Could you check a few things on this model? Use its own coordinates, in mm. A direction names the side the tool comes from. Coordinates: 2 decimals unless noted, no trailing zeros. Write each loop counter-clockwise with the first axis right and the second up, starting at its lowest first coordinate (ties: lowest second). Pieces come first, ordered by that corner, then holes. Notation, with made-up numbers: (50.5, 52.5) - (105.5, 52.5) arc R22 cw to (105.5, 86.5) - close; hole circle Ø2 at (58.5, -14.75). An arc over 180 degrees is marked (long way). Answer as a JSON object with one key per item and string values. Group by question number.
1) On a 3-axis mill with a long thin cutter (end or side, diameter ignored), from which of +Z, -Z, +X, -X, +Y, -Y can I reach the whole of each face in a straight line? I mean faces 1 (the flat face through (49, 1, -17.5)), 2 (the flat face through (20, 9, -26)), 3 (the flat face through (33, 7, 20.6)). Say none if no direction works.
2) If we section it at B-B (z = 5.35): Write out the boundary of the cut face in (x, y).
3) If we section it at C-C (z = 18.5): Write out the boundary of the cut face in (x, y).
4) If we section it at A-A (x = 34.5): Write out the boundary of the cut face in (y, z).
5) Please list where these lines run through material, in increasing order: line 1 along Z through (x, y) = (33.5, 4); line 2 along Y through (x, z) = (3.3, 5.35); line 3 along Z through (x, y) = (32, 1.25).
6) We'd pull the mould along X, two halves only. Please class faces 4 (the flat face through (2.5, 11, -7)), 5 (the flat face through (25, 11.9, -25)), 6 (the flat face through (6.5, 1, -3)): released by +X, released by -X, zero draft, split by the parting line, or undercut.
7) If we section it at D-D (y = 18.75): Write out the boundary of the cut face in (x, z), plus the area to 3 significant figures.
8) Will these pins go through, and if not, where does the flat tip stop? pin 1 Ø12 at (x, z) = (33, -2.5) entering from +Y; pin 2 Ø1.1 at (x, y) = (63, 5) entering from -Z; pin 3 Ø1.7 at (y, z) = (13, 11) entering from +X.
```python
from build123d import *

# Parameters (mm, degrees)
SKETCH1_W           = 65.5
SKETCH1_H           = 47.08
BOSS_EXTRUDE1_DEPTH = 2
BOSS_EXTRUDE2_DEPTH = 10
BOSS_EXTRUDE3_DEPTH = 3.5
SKETCH4_R           = 1.05
CUT_EXTRUDE1_DEPTH  = 73.418102709
CUT_EXTRUDE3_DEPTH  = 72.891457072
CUT_EXTRUDE8_DEPTH  = 0.5
CUT_EXTRUDE8_DRAFT  = -45
SKETCH25_W          = 3
SKETCH25_H          = 29.2
CUT_EXTRUDE10_DEPTH = 72.891457072
FILLET1_R           = 2
BOSS_EXTRUDE4_DEPTH = 10
FILLET2_R           = 1
SKETCH27_R          = 3
CUT_EXTRUDE11_DEPTH = 1
FILLET4_R           = 1
SKETCH24_R          = 7
CUT_EXTRUDE9_DEPTH  = 0.2
CUT_EXTRUDE9_DRAFT  = -45


with BuildPart() as part:
    # Sketch1 → Boss-Extrude1 (new body)
    with BuildSketch(Plane(origin=(0, 0, 0), x_dir=(1, 0, 0), z_dir=(0, 1, 0))):
        with Locations((32.75, 0)):
            Rectangle(SKETCH1_W, SKETCH1_H)
    extrude(amount=BOSS_EXTRUDE1_DEPTH)

    # Sketch2 → Boss-Extrude2 (add)
    with BuildSketch(Plane(origin=(0, 2, 0), x_dir=(1, 0, 0), z_dir=(0, 1, 0))):
        Polygon((3.5, 20.6), (62.5, 20.6), (62.5, 14.6), (65.5, 14.6), (65.5, 23.54), (0, 23.54), (0, -23.54), (65.5, -23.54), (65.5, -14.6), (62.5, -14.6), (62.5, -20.6), (3.5, -20.6), align=None)
    extrude(amount=BOSS_EXTRUDE2_DEPTH)

    # Sketch3 → Boss-Extrude3 (add)
    with BuildSketch(Plane.ZY):
        with BuildLine():
            Line((-16.65, 12), (-0.65, 12))
            Line((-0.65, 12), (-0.65, 20))
            Line((-0.65, 20), (-10.65, 20))
            ThreePointArc((-10.65, 20), (-12.771320344, 19.121320344), (-13.65, 17))
            Line((-13.65, 17), (-13.65, 15))
            ThreePointArc((-13.65, 15), (-14.528679656, 12.878679656), (-16.65, 12))
        make_face()
        with BuildLine():
            Line((-0.65, 20), (-0.65, 12))
            Line((-0.65, 12), (15.35, 12))
            ThreePointArc((15.35, 12), (13.228679656, 12.878679656), (12.35, 15))
            Line((12.35, 15), (12.35, 17))
            ThreePointArc((12.35, 17), (11.471320344, 19.121320344), (9.35, 20))
            Line((9.35, 20), (-0.65, 20))
        make_face()
    extrude(amount=-BOSS_EXTRUDE3_DEPTH)

    # Sketch4 → Cut-Extrude1 (cut, through all)
    with BuildSketch(Plane.ZY):
        with Locations((-6.65, 12.5)):
            Circle(SKETCH4_R)
        with Locations((5.35, 12.5)):
            Circle(SKETCH4_R)
    extrude(amount=-CUT_EXTRUDE1_DEPTH, mode=Mode.SUBTRACT)

    # Sketch6 → Cut-Extrude3 (cut, through all)
    with BuildSketch(Plane(origin=(0, 2, 0), x_dir=(1, 0, 0), z_dir=(0, 1, 0))):
        with BuildLine():
            Line((6.5, 15.5), (6.5, -9.096254447))
            ThreePointArc((6.5, -9.096254447), (8.036954343, -11.041913389), (10.285588719, -9.997183371))
            Line((10.285588719, -9.997183371), (22.695768518, 14.599071076))
            ThreePointArc((22.695768518, 14.599071076), (22.613391155, 16.548365908), (20.910179799, 17.5))
            Line((20.910179799, 17.5), (8.5, 17.5))
            ThreePointArc((8.5, 17.5), (7.085786438, 16.914213562), (6.5, 15.5))
        make_face()
        with BuildLine():
            Line((15.804231482, -14.599071076), (30.214411281, 13.961067028))
            ThreePointArc((30.214411281, 13.961067028), (32, 15.060138105), (33.785588719, 13.961067028))
            Line((33.785588719, 13.961067028), (48.195768518, -14.599071076))
            ThreePointArc((48.195768518, -14.599071076), (48.113391155, -16.548365908), (46.410179799, -17.5))
            Line((46.410179799, -17.5), (17.589820201, -17.5))
            ThreePointArc((17.589820201, -17.5), (15.886608845, -16.548365908), (15.804231482, -14.599071076))
        make_face()
        with BuildLine():
            Line((57.5, -9.096254447), (57.5, 15.5))
            ThreePointArc((57.5, 15.5), (56.914213562, 16.914213562), (55.5, 17.5))
            Line((55.5, 17.5), (43.089820201, 17.5))
            ThreePointArc((43.089820201, 17.5), (41.386608845, 16.548365908), (41.304231482, 14.599071076))
            Line((41.304231482, 14.599071076), (53.714411281, -9.997183371))
            ThreePointArc((53.714411281, -9.997183371), (55.963045657, -11.041913389), (57.5, -9.096254447))
        make_face()
    extrude(amount=-CUT_EXTRUDE3_DEPTH, mode=Mode.SUBTRACT)


with BuildPart() as cut_extrude8_tool:
    # Sketch23 → Cut-Extrude8 (with draft: the straight prism first)
    with BuildSketch(Plane(origin=(3.5, 0, 0), x_dir=(0, 0, -1), z_dir=(1, 0, 0))):
        with BuildLine():
            ThreePointArc((-13.5745, 12.541), (-10.3245, 9.291), (-7.0745, 12.541))
            Line((-7.0745, 12.541), (-7.0745, 22.997537045))
            Line((-7.0745, 22.997537045), (-13.5745, 22.997537045))
            Line((-13.5745, 22.997537045), (-13.5745, 12.541))
        make_face()
    extrude(amount=-CUT_EXTRUDE8_DEPTH)
    # Cut-Extrude8: the draft: its side faces are tilted about the plane it starts from
    cut_extrude8_sides = [cut_extrude8_tool.faces().sort_by_distance(p)[0] for p in [
        (3.25, 17.769268522, 7.0745),
        (3.25, 22.997537045, 10.3245),
        (3.25, 17.769268522, 13.5745),
        (3.25, 9.291, 10.3245),
    ]]
    draft(cut_extrude8_sides, Plane(origin=(3.5, 0, 0), x_dir=(0, 0, -1), z_dir=(1, 0, 0)), CUT_EXTRUDE8_DRAFT)


with BuildPart() as part_1:
    add(part.part)

    # Cut-Extrude8: cut by cut_extrude8_tool
    add(cut_extrude8_tool.part, mode=Mode.SUBTRACT)

    # Sketch25 → Cut-Extrude10 (cut, through all)
    with BuildSketch(Plane(origin=(0, 2, 0), x_dir=(1, 0, 0), z_dir=(0, 1, 0))):
        with Locations((64, 0)):
            Rectangle(SKETCH25_W, SKETCH25_H)
    extrude(amount=-CUT_EXTRUDE10_DEPTH, mode=Mode.SUBTRACT)

    # Fillet1
    fillet1_edges = [part_1.edges().sort_by_distance(p)[0] for p in [
        (65.5, 6, 14.6),
        (65.5, 6, -14.6),
        (65.5, 6, -23.54),
        (65.5, 6, 23.54),
        (0, 6, 23.54),
        (0, 6, -23.54),
    ]]
    fillet(fillet1_edges, radius=FILLET1_R)

    # Sketch26 → Boss-Extrude4 (add)
    with BuildSketch(Plane.ZY.offset(-20)):
        Polygon((-27.84, 0), (-23.54, 0), (-23.54, 2), (-25.84, 2), (-25.84, 11.9), (-23.54, 11.9), (-23.54, 12), (-20.6, 12), (-20.6, 13.9), (-27.84, 13.9), (-27.84, 12), align=None)
    extrude(amount=-BOSS_EXTRUDE4_DEPTH)

    # Fillet2
    fillet2_edges = [part_1.edges().sort_by_distance(p)[0] for p in [
        (20, 6.95, -27.84),
        (30, 1, -23.54),
        (30, 6.95, -27.84),
        (20, 1, -23.54),
    ]]
    fillet(fillet2_edges, radius=FILLET2_R)

    # Sketch27 → Cut-Extrude11 (cut)
    with BuildSketch(Plane(origin=(3.5, 0, 0), x_dir=(0, 0, -1), z_dir=(1, 0, 0))):
        with Locations((-5.35, 12.5)):
            Circle(SKETCH27_R)
        with Locations((6.65, 12.5)):
            Circle(SKETCH27_R)
    extrude(amount=-CUT_EXTRUDE11_DEPTH, mode=Mode.SUBTRACT)

    # Fillet4
    fillet4_edges = [part_1.edges().sort_by_distance(p)[0] for p in [
        (20, 12, -22.07),
        (30, 12, -22.07),
    ]]
    fillet(fillet4_edges, radius=FILLET4_R)


with BuildPart() as cut_extrude9_tool:
    # Sketch24 → Cut-Extrude9 (with draft: the straight prism first)
    with BuildSketch(Plane.XY.offset(-20.6)):
        with Locations((15.9587, 12.541)):
            Circle(SKETCH24_R)
    extrude(amount=-CUT_EXTRUDE9_DEPTH)
    # Cut-Extrude9: the draft: its side faces are tilted about the plane it starts from
    cut_extrude9_sides = [cut_extrude9_tool.faces().sort_by_distance(p)[0] for p in [
        (8.9587, 12.541, -20.7),
    ]]
    draft(cut_extrude9_sides, Plane.XY.offset(-20.6), CUT_EXTRUDE9_DRAFT)


with BuildPart() as part_2:
    add(part_1.part)

    # Cut-Extrude9: cut by cut_extrude9_tool
    add(cut_extrude9_tool.part, mode=Mode.SUBTRACT)


solid = part_2.part
```
Here are the results:
{
 "1": {"face 1": "+Y, -Y", "face 2": "-Z, -X, +Y", "face 3": "+Y"},
 "2": {"outline": "(0, 0) - (6.5, 0) - (6.5, 2) - (3.5, 2) - (3.5, 9.5) - (2.5, 9.5) - (2.5, 11.45) - (0, 11.45) - close; (0, 13.55) - (2.5, 13.55) - (2.5, 15.5) - (3.5, 15.5) - (3.5, 20) - (0, 20) - close; (12.63, 0) - (20.47, 0) - (20.47, 2) - (12.63, 2) - close; (43.53, 0) - (51.37, 0) - (51.37, 2) - (43.53, 2) - close; (57.5, 0) - (62.5, 0) - (62.5, 2) - (57.5, 2) - close"},
 "3": {"outline": "(0, 0) - (65.5, 0) - (65.5, 12) - (62.5, 12) - (62.5, 2) - (3.5, 2) - (3.5, 12) - (0, 12) - close"},
 "4": {"outline": "(0, -23.54) - (12, -23.54) - (12, -20.6) - (2, -20.6) - (2, -12.55) - (0, -12.55) - close; (0, 17.5) - (2, 17.5) - (2, 20.6) - (12, 20.6) - (12, 23.54) - (0, 23.54) - close"},
 "5": {"line 1": "z = -23.54 to -20.6, 20.6 to 23.54", "line 2": "y = 0 to 9.5, 15.5 to 20", "line 3": "z = -23.54 to -15.06, 17.5 to 23.54"},
 "6": {"face 4": "released by +X", "face 5": "zero draft", "face 6": "undercut"},
 "7": {"outline": "(0, -13.09) - (3.5, -13.09) - (3.5, 7.07) - (3, 7.57) - (3, 11.79) - (0, 11.79) - close", "area": "84.8 mm²"},
 "8": {"pin 1": "stops at y = 2", "pin 2": "stops at z = -23.54", "pin 3": "stops at x = 3"}
}
